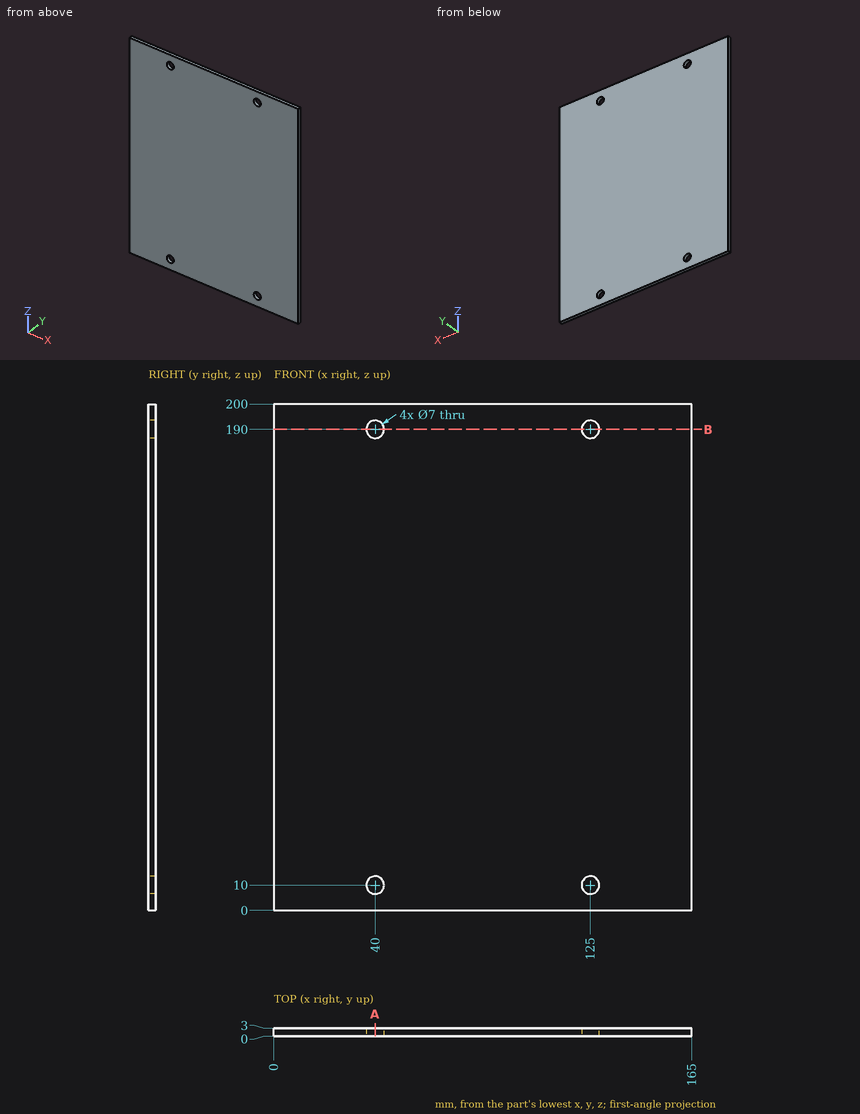
Geometry check sheet. Reference: drawing and pictorial views, mm from the part's lowest x, y, z. Coordinates: 2 decimals unless noted, no trailing zeros. Order: outer loops, then holes, each group sorted by start corner. A loop starts at its lowest first (then second) coordinate and runs counter-clockwise, first axis right, second up. Notation, with made-up numbers: (12.25, 59) -> (46.25, 59) arc R12 ccw to (46.25, 63) -> close; hole circle Ø8 at (54.25, -33). An arc over 180 degrees is marked (long way). Use CSV: the item, a comma, the result in double quotes. Start each with the question number.
Q1. Section check B-B, the plane z = 190. Record the cut outline in (x, y), and give its area (3 significant figures).
Q2. Depth check by flat-ended pin: P1, Ø6.5, axis at x = 125, z = 10, coming from the +Y side. Enter the tip coordinate at first touch or a pass-through.
Q3. Thickness scan on line 1 along Z through (x, y) = (40, 2.15). Record the ranges inside material, lowest first.
Q4. Section check A-A, the plane x = 40. Record the cut outline in (y, z).
Returned:
1,outline,"(0, 0) -> (36.5, 0) -> (36.5, 3) -> (0, 3) -> close; (43.5, 0) -> (121.5, 0) -> (121.5, 3) -> (43.5, 3) -> close; (128.5, 0) -> (165, 0) -> (165, 3) -> (128.5, 3) -> close"
1,area,"453 mm^2"
2,P1,"passes through"
3,line 1,"z = 0 to 6.5, 13.5 to 186.5, 193.5 to 200"
4,outline,"(0, 0) -> (3, 0) -> (3, 6.5) -> (0, 6.5) -> close; (0, 13.5) -> (3, 13.5) -> (3, 186.5) -> (0, 186.5) -> close; (0, 193.5) -> (3, 193.5) -> (3, 200) -> (0, 200) -> close"
